```python
from build123d import *

# Parameters (mm, degrees)
SKETCH1_W          = 1200
SKETCH1_H          = 550
BASE_FLANGE1_DEPTH = 2
EDGE_FLANGE1_DEPTH = 1200
SKETCH9_R          = 4
CUT_EXTRUDE1_DEPTH = 10
SKETCH10_R         = 110
CUT_EXTRUDE2_DEPTH = 10


# Sheet-metal steps are written as plain solids
with BuildPart() as part:
    # Base-Flange1: sheet metal written as solids
    # Sketch1 → Base-Flange1 (new body)
    with BuildSketch(Plane.XY):
        Rectangle(SKETCH1_W, SKETCH1_H)
    extrude(amount=-BASE_FLANGE1_DEPTH)

    # Edge-Flange1: sheet metal written as solids
    # Edge-Flange1 section (on a plane across the edge) → Edge-Flange1 (add)
    with BuildSketch(Plane(origin=(-600, 275.7366, -2), x_dir=(0, -1, 0), z_dir=(1, 0, 0))):
        with BuildLine():
            Line((-2, 0.7366), (-2, 33))
            Line((-2, 33), (0, 33))
            Line((0, 33), (0, 0.7366))
            ThreePointArc((0, 0.7366), (0.215745145, 0.215745145), (0.7366, 0))
            Line((0.7366, 0), (0.7366, -2))
            ThreePointArc((0.7366, -2), (-1.198468417, -1.198468417), (-2, 0.7366))
        make_face()
    extrude(amount=EDGE_FLANGE1_DEPTH)

    # Sketch9 → Cut-Extrude1 (cut)
    with BuildSketch(Plane.XZ.offset(-275.7366)):
        with Locations(Location((-550, -18.8683, 0), (0, 0, 270))):
            Circle(SKETCH9_R)
        with Locations(Location((-450, -18.8683, 0), (0, 0, 270))):
            Circle(SKETCH9_R)
        with Locations(Location((-350, -18.8683, 0), (0, 0, 270))):
            Circle(SKETCH9_R)
        with Locations(Location((-250, -18.8683, 0), (0, 0, 270))):
            Circle(SKETCH9_R)
        with Locations(Location((-150, -18.8683, 0), (0, 0, 270))):
            Circle(SKETCH9_R)
        with Locations(Location((-50, -18.8683, 0), (0, 0, 270))):
            Circle(SKETCH9_R)
        with Locations(Location((50, -18.8683, 0), (0, 0, 270))):
            Circle(SKETCH9_R)
        with Locations(Location((150, -18.8683, 0), (0, 0, 270))):
            Circle(SKETCH9_R)
        with Locations(Location((250, -18.8683, 0), (0, 0, 270))):
            Circle(SKETCH9_R)
        with Locations(Location((350, -18.8683, 0), (0, 0, 270))):
            Circle(SKETCH9_R)
        with Locations(Location((450, -18.8683, 0), (0, 0, 270))):
            Circle(SKETCH9_R)
        with Locations(Location((550, -18.8683, 0), (0, 0, 270))):
            Circle(SKETCH9_R)
    extrude(amount=-CUT_EXTRUDE1_DEPTH, mode=Mode.SUBTRACT)

    # Sketch10 → Cut-Extrude2 (cut)
    with BuildSketch(Plane.XY):
        with Locations((0, -150)):
            Circle(SKETCH10_R)
    extrude(amount=-CUT_EXTRUDE2_DEPTH, mode=Mode.SUBTRACT)


solid = part.part
```
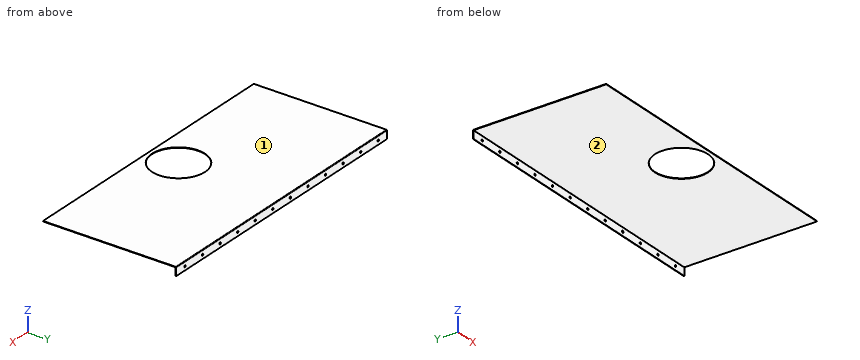
Work out the finished part from the listing and answer in its coordinate system (mm). Face numbers are marked on the shaded views. A direction names the side the tool comes from. Give positions to 0.01 mm unless a question says otherwise; leave off trailing zeros. Write each loop counter-clockwise with the first axis right and the second up, starting at its lowest first coordinate (ties: lowest second). Pieces come first, ordered by that corner, then holes. Notation, with made-up numbers: (21.25, 57.5) -> (44.25, 57.5) arc R37 cw to (44.25, 93.5) -> close; hole circle Ø4 at (-16.5, -31.75). An arc over 180 degrees is marked (long way). Write item = value, one per line.
Q1. Consider line 1 along Z through (x, y) = (-450, 276); line 2 along Y through (x, z) = (525.5, -32.5); line 3 along Z through (x, y) = (27, 26). Determine where each line is inside the solid, lowest interval first.
Computed values:
line_1 = -35 to -22.87, -14.87 to -0.19
line_2 = 275.74 to 277.74
line_3 = -2 to 0
Q2. Section B-B on x = 174 is taken. Determine the outline of the cut face in (y, z).
Computed values:
outline = (-275, -2) -> (275, -2) arc R0.74 cw to (275.74, -2.74) -> (275.74, -35) -> (277.74, -35) -> (277.74, -2.74) arc R2.74 ccw to (275, 0) -> (-275, 0) -> close
Q3. Section C-C on y = 186 is taken. Determine the outline of the cut face in (x, z).
Computed values:
outline = (-600, -2) -> (600, -2) -> (600, 0) -> (-600, 0) -> close
Q4. Section A-A on y = -81 is taken. Determine the outline of the cut face in (x, z).
Computed values:
outline = (-600, -2) -> (-85.67, -2) -> (-85.67, 0) -> (-600, 0) -> close; (85.67, -2) -> (600, -2) -> (600, 0) -> (85.67, 0) -> close
Q5. A tool of negligible diameter and unlimited length cuts with its end or side. For the marked faces 1 and 2, from which of +Z, -Z, +X, -X, +Y, -Y can it reach the whole face along a straight path? Write none if from no direction.
Computed values:
face_1 = +Z, +X, -X, +Y, -Y
face_2 = -Z, +X, -X, -Y
Q6. Flat-ended cylindrical pins translate along their axes: pin 1 Ø2 at (x, y) = (129.5, 88.5) entering from -Z; pin 2 Ø7 at (x, z) = (-250, -18.87) entering from -Y; pin 3 Ø13 at (x, z) = (50, -18.87) entering from -Y; pin 4 Ø9 at (x, z) = (450, -18.87) entering from +Y. Find the tip coordinate at first contact, or state that the pin passes through.
Computed values:
pin_1 = -2
pin_2 = through
pin_3 = 275.74
pin_4 = 277.74
